Autodesk Inventor part; units mm, degrees
ref_plane "YZ Plane" through (0, 0, 0) normal (1, 0, 0) x (0, 1, 0)
ref_plane "XZ Plane" through (0, 0, 0) normal (0, 1, 0) x (-1, 0, 0)
ref_plane "XY Plane" through (0, 0, 0) normal (0, 0, 1) x (1, 0, 0)
sketch "Sketch1" plane through (0, 0, 0) normal (0, 1, 0) x (-1, 0, 0)
  line L0 (-12.7, 12.7) -> (12.7, 12.7)
  line L1 (12.7, 12.7) -> (12.7, -12.7)
  line L2 (12.7, -12.7) -> (-12.7, -12.7)
  line L3 (-12.7, -12.7) -> (-12.7, 12.7)
  line L4 (-12.7, 12.7) -> (12.7, -12.7) construction
  line L5 (12.7, 12.7) -> (-12.7, -12.7) construction
  point P0 (0, 0)
  dimension "d0" = 25.4
  dimension "d1" = 25.4
extrude "Extrusion1" add sketch "Sketch1" along normal blind 3.175
sketch "Sketch2" plane through (0, 3.175, 0) normal (0, 1, 0) x (1, 0, 0)
  line L0 (7.4295, -8.1915) -> (-7.4295, -8.1915)
  line L1 (-7.4295, -8.1915) -> (-7.4295, 8.1915)
  line L2 (-7.4295, 8.1915) -> (7.4295, 8.1915)
  line L3 (7.4295, 8.1915) -> (7.4295, -8.1915)
  line L4 (7.4295, -8.1915) -> (-7.4295, 8.1915) construction
  line L5 (-7.4295, -8.1915) -> (7.4295, 8.1915) construction
  point P0 (0, 0)
  dimension "d4" = 14.859
  dimension "d5" = 16.383
extrude "Extrusion2" cut sketch "Sketch2" against normal through all
sketch "Sketch3" plane through (0, 3.175, 0) normal (0, 1, 0) x (1, 0, 0)
  line L0 (-7.4295, -8.1915) -> (-7.4295, 8.1915)
  line L1 (-7.4295, -8.1915) -> (-12.5095, -8.1915)
  line L2 (-12.5095, -8.1915) -> (-12.5095, 8.1915)
  line L3 (-12.5095, 8.1915) -> (-7.4295, 8.1915)
  line L4 (-7.4295, 8.1915) -> (-7.4295, -8.1915)
  line L5 (-12.5095, -8.1915) -> (9.9695, -8.1915)
  line L6 (9.9695, -8.1915) -> (9.9695, -10.7315)
  line L7 (9.9695, -10.7315) -> (-12.5095, -10.7315)
  line L8 (-12.5095, -10.7315) -> (-12.5095, -8.1915)
  line L9 (7.4295, 8.1915) -> (7.4295, -8.1915)
  line L10 (-12.5095, 8.1915) -> (9.9695, 8.1915)
  line L11 (9.9695, 8.1915) -> (9.9695, 10.7315)
  line L12 (9.9695, 10.7315) -> (-12.5095, 10.7315)
  line L13 (-12.5095, 10.7315) -> (-12.5095, 8.1915)
  point P0 (0, 0)
  point P1 (-9.9695, 8.1915)
  point P2 (9.9695, -9.4615)
  point P3 (9.9695, 9.4615)
  dimension "d11" = 2.54
  dimension "d12" = 2.54
  dimension "d13" = 2.54
  dimension "d14" = 5.08
extrude "Extrusion3" add sketch "Sketch3" along normal blind 6.985 contours L1 L2 L3 L0 | L5 L6 L7 L8 L1 | L3 L13 L12 L11 L10
sketch "Sketch4" plane through (0, 10.16, 0) normal (0, 1, 0) x (1, 0, 0)
  line L0 (-7.4295, -8.1915) -> (-7.4295, 8.1915) construction
  line L1 (-7.4295, -3.81) -> (-9.7155, -3.81) construction
  line L2 (-9.7155, -3.81) -> (-9.7155, 3.81) construction
  line L3 (-9.7155, 3.81) -> (-7.4295, 3.81) construction
  line L4 (-7.4295, 3.81) -> (-7.4295, -3.81) construction
  circle A0 centre (-10.4775, 0) radius 1.143 construction
  circle A1 centre (-10.4775, 0) radius 0.9525
  point P0 (0, 0)
  point P1 (-7.4295, 0)
  point P2 (-9.7155, 0)
  dimension "d15" = 2.286
  dimension "d16" = 7.62
  dimension "d17" = 2.286
  dimension "d18" = 1.905
  dimension "d21" = 0.762
extrude "Extrusion4" cut sketch "Sketch4" against normal blind 6.35
properties part number "RJ45Insert"
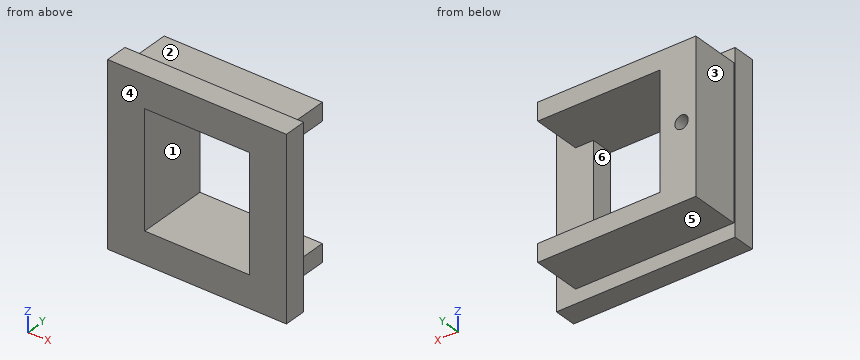
CAD build for the part. Positions are in the model's coordinates, mm. Face numbers are marked on the shaded views. A direction names the side the tool comes from. Give positions to 0.01 mm unless a question says otherwise; leave off trailing zeros. Write each loop counter-clockwise with the first axis right and the second up, starting at its lowest first coordinate (ties: lowest second). Pieces come first, ordered by that corner, then holes. Notation, with made-up numbers: (30.5, -4) -> (87.5, -4) arc R14 cw to (87.5, 4) -> close; hole circle Ø7 at (-12.75, 32). An arc over 180 degrees is marked (long way). Write each question's results on one line, items separated by ' | '.
1. Cut at C-C, the plane y = 4.5. Write the cut outline in (x, z) (1 decimal), then the cut area to 3 significant figures.
Geometry check:
outline: (-12.5, -10.7) -> (10, -10.7) -> (10, -8.2) -> (-7.4, -8.2) -> (-7.4, 8.2) -> (10, 8.2) -> (10, 10.7) -> (-12.5, 10.7) -> close; hole circle Ø1.9 at (-10.5, 0) | area: 195 mm²
2. Wall check: probe 1 along X at (y, z) = (5.5, 0) (1 decimal); probe 2 along X at (y, z) = (1, 8); probe 3 along Z at (x, y) = (4, 3.25). Give the ranges that are in metal, low to high. Write a range as [from, to].
Geometry check:
probe 1: [-12.5, -11.4], [-9.5, -7.4] | probe 2: [-12.7, -7.43], [7.43, 12.7] | probe 3: [-10.73, -8.19], [8.19, 10.73]
3. Two-plate mould, pull along Z, no slides. Class the marked faces 4, 5 and 6: pulls with the +Z half, pulls with the -Z half, needs draft (parallel to the pull), parting line crosses it, or undercut.
Geometry check:
face 4: needs draft | face 5: pulls with the -Z half | face 6: undercut
4. Cut at B-B, the plane x = 0.5. Write the cut outline in (y, z) (1 decimal), then the cut area to 3 significant figures.
Geometry check:
outline: (0, -12.7) -> (3.2, -12.7) -> (3.2, -10.7) -> (10.2, -10.7) -> (10.2, -8.2) -> (0, -8.2) -> close; (0, 8.2) -> (10.2, 8.2) -> (10.2, 10.7) -> (3.2, 10.7) -> (3.2, 12.7) -> (0, 12.7) -> close | area: 64.1 mm²
5. Which spindle directions (+Z, -Z, +X, -X, +Y, -Y) get a long thin tool onto all of the face, cutting with end or side? Do the marked faces 1, 2 and 3. Say none if no direction does.
Geometry check:
face 1: +Y, -Y | face 2: +Z, +X, -X, +Y | face 3: +Z, -Z, -X, +Y
6. Drop flat-ended pins along their axis: P1, Ø5.5, axis at x = 1.5, y = 7, coming from the +Z side; P2, Ø1.5, axis at x = -11, z = 0, coming from the +Y side; P3, Ø2, axis at y = 6.5, z = -5.5, coming from the -X side; P4, Ø3, axis at y = 5, z = 9, coming from the +X side. Give the stop position or say it passes through.
Geometry check:
P1: z = 10.73 | P2: y = 10.16 | P3: x = -12.51 | P4: x = 9.97
